Here's how the part is built. I have some questions about the finished solid (model axes, mm). A direction names the side the tool comes from. Round coordinates to 2 decimals unless told otherwise and drop trailing zeros. Write each loop counter-clockwise with the first axis right and the second up, starting at its lowest first coordinate (ties: lowest second). Pieces come first, ordered by that corner, then holes. Notation, with made-up numbers: (36.25, 56) -> (93.25, 56) arc R24 ccw to (93.25, 70) -> close; hole circle Ø4 at (-15, 31). An arc over 180 degrees is marked (long way). Answer as CSV lines item,"result".
Autodesk Inventor part; units mm, degrees
ref_plane "YZ Plane" through (0, 0, 0) normal (1, 0, 0) x (0, 1, 0)
ref_plane "XZ Plane" through (0, 0, 0) normal (0, 1, 0) x (-1, 0, 0)
ref_plane "XY Plane" through (0, 0, 0) normal (0, 0, 1) x (1, 0, 0)
sketch "Sketch1" plane through (0, 0, 0) normal (0, 0, 1) x (1, 0, 0)
  circle A0 centre (0, 0) radius 40
  dimension "d0" = 80
extrude "Extrusion1" add sketch "Sketch1" along normal blind 22.5
sketch "Sketch2" plane through (0, 0, 22.5) normal (0, 0, 1) x (1, 0, 0)
  point P0 (0, 0)
  point P1 (0, 35)
  dimension "d3" = 35
hole "Hole1" at (0, 35, 22.5) direction (0, 0, -1) diameter 4.3 end through all counterbore diameter 10.59 counterbore depth 5
chamfer "Chamfer1" distance 2 distance2 3 2 edges at (-27.6179, -28.9353, 22.5) (28.9353, 27.6179, 22.5) measured on face at (-2.7418, -16.4668, 22.5)
pattern_circular "Circular Pattern1" count 6 over 360 about axis through (0, 0, 0) along (0, 0, 1) of "Hole1"
sketch "Sketch3" plane through (0, 0, 0) normal (0, 0, -1) x (-1, 0, 0)
  circle A0 centre (0, 0) radius 29.1
  dimension "d17" = 58.2
extrude "Extrusion2" cut sketch "Sketch3" against normal through all
ref_plane "Work Plane1" through (0, 0, 10.5) normal (0, 0, -1) x (-1, 0, 0)
sketch "Sketch4" plane through (0, 0, 10.5) normal (0, 0, -1) x (-1, 0, 0)
  circle A0 centre (0, 0) radius 29.5
  circle A1 centre (0, 0) radius 26.5
  dimension "d21" = 53
  dimension "d22" = 59
extrude "Extrusion3" add sketch "Sketch4" against normal blind 3
sketch "Sketch5" plane through (0, 0, 22.5) normal (0, 0, 1) x (1, 0, 0)
  arc A0 (33.6722, 21.5913) -> (1.8625, 39.9566) centre (0, 0) ccw
  line L0 (0, 0) -> (40, 0) construction
  line L1 (21.3532, 22.5799) -> (24.5138, 27.0811)
  line L2 (24.5138, 27.0811) -> (17.1481, 32.253)
  line L3 (17.1481, 32.253) -> (13.9876, 27.7518)
  line L4 (13.9876, 27.7518) -> (21.3532, 22.5799)
  line L5 (21.3532, 22.5799) -> (17.1481, 32.253) construction
  line L6 (24.5138, 27.0811) -> (13.9876, 27.7518) construction
  line L7 (16.4837, 25.9991) -> (19.6443, 30.5003)
  line L8 (22.0585, 28.8051) -> (18.898, 24.3039)
  line L9 (14.3755, 28.3042) -> (16.7602, 31.7005)
  line L10 (16.7602, 31.7005) -> (19.2564, 29.9479)
  line L11 (19.2564, 29.9479) -> (16.8716, 26.5515)
  line L12 (16.8716, 26.5515) -> (14.3755, 28.3042)
  line L13 (19.2507, 27.4165) -> (15.5679, 30.0024)
  line L14 (16.8716, 26.5515) -> (16.7602, 31.7005)
  line L15 (14.3755, 28.3042) -> (19.2564, 29.9479)
  line L16 (0, 0) -> (16.8159, 29.126)
  line L17 (0, 0) -> (19.2507, 27.4165)
  point P0 (16.8716, 26.5515)
  dimension "d26" = 9
  dimension "d27" = 5.5
  dimension "d29" = 33.5
  dimension "d30" = 3.05
  dimension "d36" = 3
  dimension "d41" = 4.15
  dimension "d42" = 60
extrude "Extrusion4" cut sketch "Sketch5" against normal blind 1.75 contours L4 L17 L13 L7 L2 L8 | L4 L7 L13 L17 | L15 L14 L10 | L7 L13 L15 | L14 L13 L7 | L12 L16 L14 | L14 L13 L3 | L15 L3 L13 | L16 L12 L15
extrude "Extrusion7" cut sketch "Sketch5" against normal through all contours L4 L8 L2 L1
properties part number "Ring Cover Top"
Item 1: Suppose I cut it at B-B, the plane x = 0. List the corners of the cut face in (y, z) for me (3 decimals), then the cut area to 3 significant figures.
Results found:
outline,"(-40, 0) -> (-37.15, 0) -> (-37.15, 17.5) -> (-40, 17.5) -> close; (-32.85, 0) -> (-29.1, 0) -> (-29.1, 10.5) -> (-26.5, 10.5) -> (-26.5, 13.5) -> (-29.1, 13.5) -> (-29.1, 22.5) -> (-29.705, 22.5) -> (-29.705, 17.5) -> (-32.85, 17.5) -> close; (26.5, 10.5) -> (29.1, 10.5) -> (29.1, 0) -> (32.85, 0) -> (32.85, 17.5) -> (29.705, 17.5) -> (29.705, 22.5) -> (29.1, 22.5) -> (29.1, 13.5) -> (26.5, 13.5) -> close; (37.15, 0) -> (40, 0) -> (40, 17.5) -> (37.15, 17.5) -> close"
area,"253 mm²"
Item 2: If we mould it in two halves opening along X, with no side actions, what happens to faces 1 (the conical face through (19.171, 33.723, 21.312)), 2 (the cylindrical face through (-25.83, -14.68, 19.96)), 3 (the flat face through (20.5, 26.586, 10.52)), 4 (the conical face through (-19.62, 33.464, 21.312))? For each: pulls with the +X half, pulls with the -X half, needs draft (parallel to the pull), parting line crosses it, or undercut.
Results found:
face 1,"pulls with the +X half"
face 2,"undercut"
face 3,"undercut"
face 4,"pulls with the -X half"
Item 3: Will these pins go through, and if not, where does the flat tip stop? pin 1 (1.5 mm diameter, centred on y = -4.5, z = 7.5, fed in from -X); pin 2 (5.5 mm diameter, centred on x = -32.5, y = 16.5, fed in from +Z); pin 3 (3 mm diameter, centred on y = -6, z = 7.5, fed in from -X).
Results found:
pin 1,"stops at x = -39.82"
pin 2,"stops at z = 17.5"
pin 3,"stops at x = -39.75"
Item 4: I need wall thicknesses on L1, parallel to X at y = -1, z = 16; L2, parallel to Y at x = 0, z = 19.75 (3 decimals); L3, parallel to Y at x = -29.5, z = 4.25. Which ranges of each line are inside material? Lowest first, please.
Results found:
L1,"x = -39.99 to -29.08, 29.08 to 39.99"
L2,"y = -29.705 to -29.1, 29.1 to 29.705"
L3,"y = -27.01 to -19.49, -15.51 to 15.51, 19.49 to 27.01"
Item 5: Suppose I cut it at C-C, the plane z = 16.5. State how many separate pieces and enclosed holes the cut face has, then the cut area to 3 significant figures.
Results found:
separate pieces,"1"
enclosed holes,"8"
area,"2,260 mm²"
Item 6: For faces 5 (the conical face through (39, 0, 21)), 6 (the flat face through (26, 7, 13.5)), 7 (the cylindrical face through (3.788, 28.852, 5.176)), 8 (the flat face through (22.91, 24.8, 11.41)), 9 (the conical face through (-39, 0, 21)), which set-ups out of +Z, -Z, +X, -X, +Y, -Y let a thin tool reach every point of the face, with its end or its side?
Results found:
face 5,"+Z, +X"
face 6,"+Z"
face 7,"-Z"
face 8,"+Z, -Z"
face 9,"+Z, -X"
Item 7: Suppose I cut it at A-A, the plane y = 0. List the corners of the cut face in (x, z) for me.
Results found:
outline,"(-40, 0) -> (-29.1, 0) -> (-29.1, 10.5) -> (-26.5, 10.5) -> (-26.5, 13.5) -> (-29.1, 13.5) -> (-29.1, 22.5) -> (-38, 22.5) -> (-40, 19.5) -> close; (26.5, 10.5) -> (29.1, 10.5) -> (29.1, 0) -> (40, 0) -> (40, 19.5) -> (38, 22.5) -> (29.1, 22.5) -> (29.1, 13.5) -> (26.5, 13.5) -> close"
